Can you work these out from the drawing? Everything is in mm from the part's minimum corner. Coordinates: 2 decimals unless noted, no trailing zeros. Loops run counter-clockwise (first coordinate to the right, second up) from the corner with the lowest first, then second, coordinate; pieces in that order, holes last.
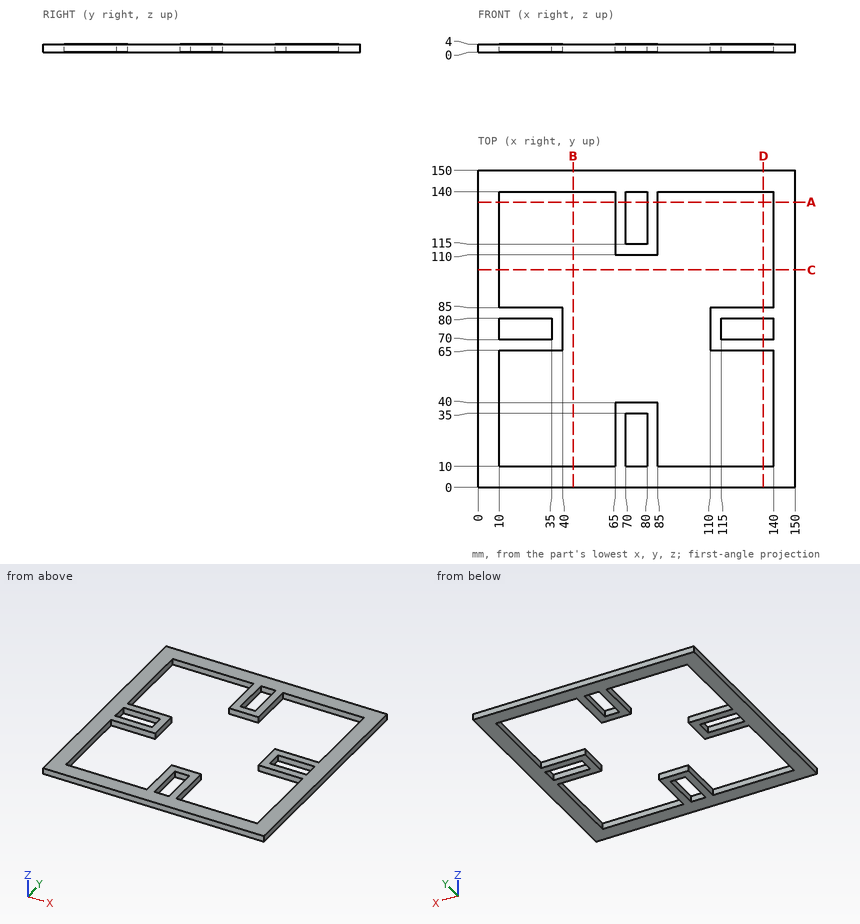
1. I want a section at B-B (x = 45). Please give me the cut outline in (y, z), then the cut area to 3 significant figures.
2. I need wall thicknesses on line 1 along Y through (x, z) = (14.5, 2.9); line 2 along X through (y, z) = (79, 1.2); line 3 along X through (y, z) = (111.5, 3). Which ranges of each line are inside material? Lowest first, please.
3. I want a section at A-A (y = 135). Please give me the cut outline in (x, z), then the cut area to 3 significant figures.
Response values:
1. outline: (0, 0) - (10, 0) - (10, 4) - (0, 4) - close; (140, 0) - (150, 0) - (150, 4) - (140, 4) - close
1. area: 80.0 mm2
2. line 1: y = 0 to 10, 65 to 70, 80 to 85, 140 to 150
2. line 2: x = 0 to 10, 35 to 40, 110 to 115, 140 to 150
2. line 3: x = 0 to 10, 65 to 85, 140 to 150
3. outline: (0, 0) - (10, 0) - (10, 4) - (0, 4) - close; (65, 0) - (70, 0) - (70, 4) - (65, 4) - close; (80, 0) - (85, 0) - (85, 4) - (80, 4) - close; (140, 0) - (150, 0) - (150, 4) - (140, 4) - close
3. area: 120 mm2
